```python
from build123d import *

# Parameters (mm, degrees)
F0_W     = 70.8
F0_H     = 145.75
F1_DEPTH = 6.26
F2_R     = 3.12999


# Not quite as in the source:
# - a fillet or chamfer is up to 0.001 mm smaller than in the source, because OpenCascade refuses the exact size


with BuildPart() as f1:
    # F0 (on Top) → F1 (new body)
    with BuildSketch(Plane.XY):
        Rectangle(F0_W, F0_H)
        with BuildLine():
            Line((-34.9, -69.245), (-34.9, 69.245))
            ThreePointArc((-34.9, 69.245), (-33.9832442251, 71.4582442251), (-31.77, 72.375))
            Line((-31.77, 72.375), (31.77, 72.375))
            ThreePointArc((31.77, 72.375), (33.9832442251, 71.4582442251), (34.9, 69.245))
            Line((34.9, 69.245), (34.9, -69.245))
            ThreePointArc((34.9, -69.245), (33.9832442251, -71.4582442251), (31.77, -72.375))
            Line((31.77, -72.375), (-31.77, -72.375))
            ThreePointArc((-31.77, -72.375), (-33.9832442251, -71.4582442251), (-34.9, -69.245))
        make_face(mode=Mode.SUBTRACT)
        with BuildLine():
            ThreePointArc((-31.77, 72.375), (-33.9832442251, 71.4582442251), (-34.9, 69.245))
            Line((-34.9, 69.245), (-34.9, -69.245))
            ThreePointArc((-34.9, -69.245), (-33.9832442251, -71.4582442251), (-31.77, -72.375))
            Line((-31.77, -72.375), (31.77, -72.375))
            ThreePointArc((31.77, -72.375), (33.9832442251, -71.4582442251), (34.9, -69.245))
            Line((34.9, -69.245), (34.9, 69.245))
            ThreePointArc((34.9, 69.245), (33.9832442251, 71.4582442251), (31.77, 72.375))
            Line((31.77, 72.375), (-31.77, 72.375))
        make_face()
    extrude(amount=-F1_DEPTH)

    # F2 (radius 3.13 in the source; OpenCascade refuses exactly that, so slightly less here)
    f2_edges = [f1.edges().sort_by_distance(p)[0] for p in [
        (35.4, 0, 0),
        (0, 72.875, 0),
        (-35.4, 0, 0),
        (0, -72.875, 0),
        (35.4, 0, -6.26),
        (0, 72.875, -6.26),
        (-35.4, 0, -6.26),
        (0, -72.875, -6.26),
        (35.4, -72.875, -3.13),
        (-35.4, -72.875, -3.13),
        (-35.4, 72.875, -3.13),
        (35.4, 72.875, -3.13),
    ]]
    fillet(f2_edges, radius=F2_R)


solid = f1.part
```
Geometry check sheet. Reference: the model listing, model coordinates, mm. Coordinates: 2 decimals unless noted, no trailing zeros. Write each loop counter-clockwise with the first axis right and the second up, starting at its lowest first coordinate (ties: lowest second). Pieces come first, ordered by that corner, then holes. Notation, with made-up numbers: M 21,-6.5 L 29,-6.5 A26 cw 29,21.5 Z; hole C -39,72.5 d1. An arc over 180 degrees is marked long. Answer as a JSON object with one key per item and string values.
1. Go/stop test with a flat-tipped pin: pin 1 Ø1.5 at (y, z) = (21.5, -1) entering from +X. Record where the tip stops, or that it passes through.
Answers below:
{"pin 1": "stops at x = 35.08"}
2. Section check B-B, the plane z = -1. Enter the section's corners in (x, y) (3 decimals), plus the area to 3 significant figures.
Answers below:
{"outline": "M -34.563,-69.745 A2.293 ccw -32.27,-72.038 L 32.27,-72.038 A2.293 ccw 34.563,-69.745 L 34.563,69.745 A2.293 ccw 32.27,72.038 L -32.27,72.038 A2.293 ccw -34.563,69.745 Z", "area": "9,960 mm²"}
3. Scan lines: L1, parallel to X at y = 58.5, z = -3.25; L2, parallel to Y at x = -11.5, z = -3; L3, parallel to Y at x = 2.5, z = -4.75. Record each from-to range of solid material in increasing order.
Answers below:
{"L1": "x = -35.4 to 35.4", "L2": "y = -72.87 to 72.87", "L3": "y = -72.42 to 72.42"}
